Job drawing, mm, ordinate dimensions from the low corner. One solid piece. A direction names the side the tool comes from. Round coordinates to 2 decimals unless told otherwise and drop trailing zeros. Loops run counter-clockwise (first coordinate to the right, second up) from the corner with the lowest first, then second, coordinate; pieces in that order, holes last. Notation, with made-up numbers: M -40,84 L 9,84 A17 ccw 9,100 Z; hole C 9.5,-13.5 d1. An arc over 180 degrees is marked long. Use a Markdown table: item, result. Add a question column.
(1) Band-saw the part on B-B, the plane y = 11.5. Write the cut outline in (x, z).
(2) Two-plate mould, pull along Z, no slides. Class the marked faces 3, 4 and 5: released by +Z, released by -Z, zero draft, split by the parting line, or undercut.
(3) Band-saw the part on A-A, the plane z = 3. Write the cut outline in (x, y).
(4) Band-saw the part on D-D, the plane z = 5.6. Write the cut outline in (x, y).
(5) Wall check: L1, parallel to X at y = 15.75, z = 4.4; L2, parallel to Y at x = 6, z = 4.95; L3, parallel to Z at x = 11.45, y = 6.25. Give the ranges that are in metal, low to high.
(6) Band-saw the part on C-C, the plane x = 11.45. Write the cut outline in (y, z), and give its area (3 significant figures).
(7) Which spindle directions (+Z, -Z, +X, -X, +Y, -Y) get a long thin tool onto all of the face, cutting with end or side? Do the marked faces 1 and 2. Say none if no direction does.
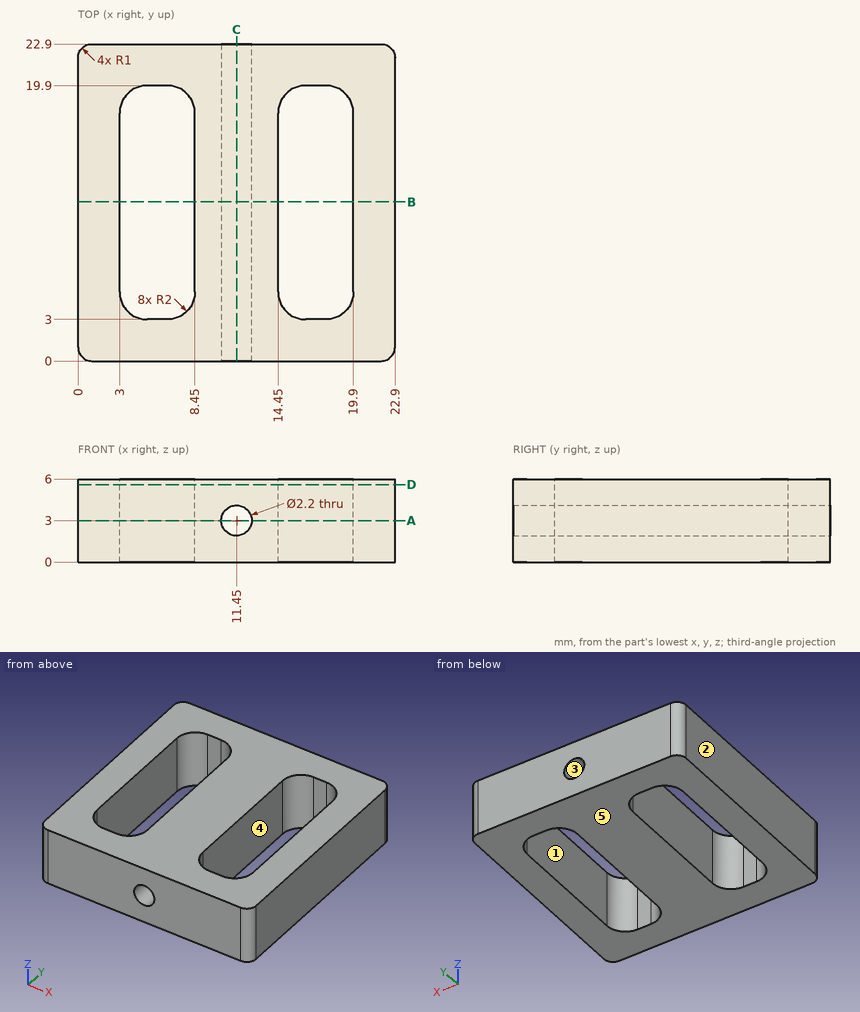
Return value:
| question | item | result |
|---|---|---|
| 1 | outline | M 0,0 L 3,0 L 3,6 L 0,6 Z; M 8.45,0 L 14.45,0 L 14.45,6 L 8.45,6 Z; M 19.9,0 L 22.9,0 L 22.9,6 L 19.9,6 Z; hole C 11.45,3 d2.2 |
| 2 | face 3 | undercut |
| 2 | face 4 | zero draft |
| 2 | face 5 | released by -Z |
| 3 | outline | M 0,1 A1 ccw 1,0 L 10.35,0 L 10.35,22.9 L 1,22.9 A1 ccw 0,21.9 Z; M 12.55,0 L 21.9,0 A1 ccw 22.9,1 L 22.9,21.9 A1 ccw 21.9,22.9 L 12.55,22.9 Z; hole M 3,5 A2 ccw 5,3 L 6.45,3 A2 ccw 8.45,5 L 8.45,17.9 A2 ccw 6.45,19.9 L 5,19.9 A2 ccw 3,17.9 Z; hole M 14.45,5 A2 ccw 16.45,3 L 17.9,3 A2 ccw 19.9,5 L 19.9,17.9 A2 ccw 17.9,19.9 L 16.45,19.9 A2 ccw 14.45,17.9 Z |
| 4 | outline | M 0,1 A1 ccw 1,0 L 21.9,0 A1 ccw 22.9,1 L 22.9,21.9 A1 ccw 21.9,22.9 L 1,22.9 A1 ccw 0,21.9 Z; hole M 3,5 A2 ccw 5,3 L 6.45,3 A2 ccw 8.45,5 L 8.45,17.9 A2 ccw 6.45,19.9 L 5,19.9 A2 ccw 3,17.9 Z; hole M 14.45,5 A2 ccw 16.45,3 L 17.9,3 A2 ccw 19.9,5 L 19.9,17.9 A2 ccw 17.9,19.9 L 16.45,19.9 A2 ccw 14.45,17.9 Z |
| 5 | L1 | 0 to 3, 8.45 to 14.45, 19.9 to 22.9 |
| 5 | L2 | 0 to 3, 19.9 to 22.9 |
| 5 | L3 | 0 to 1.9, 4.1 to 6 |
| 6 | outline | M 0,0 L 22.9,0 L 22.9,1.9 L 0,1.9 Z; M 0,4.1 L 22.9,4.1 L 22.9,6 L 0,6 Z |
| 6 | area | 87.0 mm^2 |
| 7 | face 1 | +Z, -Z |
| 7 | face 2 | +Z, -Z, -X, +Y, -Y |
